```python
from build123d import *

# Parameters (mm, degrees)
SKETCH1_W           = 10
SKETCH1_H           = 10
BOSS_EXTRUDE1_DEPTH = 2
SKETCH2_R           = 1.55
SKETCH2_R_2         = 1.6
SKETCH2_R_3         = 0.5
SKETCH2_W           = 1.85
SKETCH2_H           = 1.85
SKETCH2_W_2         = 1.95
SKETCH2_H_2         = 1.95
SKETCH2_W_3         = 1.9
SKETCH2_H_3         = 1.9
CUT_EXTRUDE1_DEPTH  = 10
FILLET1_R           = 2


with BuildPart() as part:
    # Sketch1 → Boss-Extrude1 (new body)
    with BuildSketch(Plane(origin=(0, 0, 0), x_dir=(1, 0, 0), z_dir=(0, 1, 0))):
        with Locations((-46.016664058, -38.292528072)):
            Rectangle(SKETCH1_W, SKETCH1_H)
    extrude(amount=BOSS_EXTRUDE1_DEPTH)

    # Sketch2 → Cut-Extrude1 (cut)
    with BuildSketch(Plane(origin=(0, 2, 0), x_dir=(1, 0, 0), z_dir=(0, 1, 0))):
        with Locations(Location((-48.08551258, -40.164750495, 0), (0, 0, 270))):
            Circle(SKETCH2_R)
        with Locations(Location((-43.742640476, -40.164750495, 0), (0, 0, 270))):
            Circle(SKETCH2_R_2)
        with Locations(Location((-49.709815138, -37.736845618, 0), (0, 0, 270))):
            Circle(SKETCH2_R_3)
        with Locations((-48.955794355, -35.478207728)):
            Rectangle(SKETCH2_W, SKETCH2_H)
        with Locations((-43.041207223, -35.394011884)):
            Rectangle(SKETCH2_W_2, SKETCH2_H_2)
        with Locations((-46.016664058, -35.479919958)):
            Rectangle(SKETCH2_W_3, SKETCH2_H_3)
    extrude(amount=-CUT_EXTRUDE1_DEPTH, mode=Mode.SUBTRACT)

    # Fillet1
    fillet1_edges = [part.edges().sort_by_distance(p)[0] for p in [
        (-51.016664058, 1, 33.292528072),
        (-41.016664058, 1, 33.292528072),
        (-41.016664058, 1, 43.292528072),
        (-51.016664058, 1, 43.292528072),
    ]]
    fillet(fillet1_edges, radius=FILLET1_R)


solid = part.part
```
Geometry: final body of the model. Coordinates: model frame, mm. A direction names the side the tool comes from. Round coordinates to 2 decimals unless told otherwise and drop trailing zeros. Order: outer loops, then holes, each group sorted by start corner. A loop starts at its lowest first (then second) coordinate and runs counter-clockwise, first axis right, second up. Notation, with made-up numbers: (66.25, -39.75) - (118.25, -39.75) arc R32 ccw to (118.25, -0.75) - close; hole circle Ø10 at (86.5, 88). An arc over 180 degrees is marked (long way). Use CSV: the item, a comma, the result in double quotes. Start each with the question number.
Q1. Material intervals for line 1 along X through (y, z) = (1.55, 36); line 2 along Z through (x, y) = (-46.75, 0.7); line 3 along Z through (x, y) = (-43.5, 0.5), sorted ascending. Write a range as from..to.
Q2. Section query C-C (z = 37.5). Return loops of the section in (x, y), and give its area (3 significant figures).
Q3. Section query D-D (y = 0.6). Return loops of the section in (x, z), and give its area (3 significant figures).
Q4. Access query for faces 4 (the face through (-49, 1, 36.403)), 5 (the face through (-46, 0, 38)). Directions: +Z, -Z, +X, -X, +Y, -Y. A direction counts if a zero-diameter tool reaches every point of the face in a straight line with its end or side. Return the directions, or none.
Q5. Section query B-B (x = -50). Return loops of the section in (y, z).
Q6. Mould query, pull axis X, two halves, no side actions, for faces 1 (the face through (-41.618, 1.014, 42.722)), 2 (the face through (-43, 1, 36.369)), 3 (the face through (-46, 1, 43.293)). Classes: +X half, -X half, draft (parallel to the pull), parting line (faces both ways), or undercut.
Q7. Section query A-A (z = 35.5). Return loops of the section in (x, y), and give its area (3 significant figures).
Result set:
1,line 1,"x = -51.02..-49.88, -48.03..-46.97, -45.07..-44.02, -42.07..-41.02"
1,line 2,"z = 33.29..34.53, 36.43..39.38, 40.95..43.29"
1,line 3,"z = 33.29..34.42, 36.37..38.58, 41.75..43.29"
2,outline,"(-51.02, 0) - (-50.15, 0) - (-50.15, 2) - (-51.02, 2) - close; (-49.27, 0) - (-41.02, 0) - (-41.02, 2) - (-49.27, 2) - close"
2,area,"18.2 mm2"
3,outline,"(-51.02, 35.29) arc R2 ccw to (-49.02, 33.29) - (-43.02, 33.29) arc R2 ccw to (-41.02, 35.29) - (-41.02, 41.29) arc R2 ccw to (-43.02, 43.29) - (-49.02, 43.29) arc R2 ccw to (-51.02, 41.29) - close; hole circle Ø1 at (-49.71, 37.74); hole (-49.88, 34.55) - (-48.03, 34.55) - (-48.03, 36.4) - (-49.88, 36.4) - close; hole circle Ø3.1 at (-48.09, 40.16); hole (-46.97, 34.53) - (-45.07, 34.53) - (-45.07, 36.43) - (-46.97, 36.43) - close; hole circle Ø3.2 at (-43.74, 40.16); hole (-44.02, 34.42) - (-42.07, 34.42) - (-42.07, 36.37) - (-44.02, 36.37) - close"
3,area,"69.4 mm2"
4,face 4,"+Y, -Y"
4,face 5,"+Z, -Z, +X, -X, -Y"
5,outline,"(0, 33.55) - (2, 33.55) - (2, 37.33) - (0, 37.33) - close; (0, 38.14) - (2, 38.14) - (2, 43.03) - (0, 43.03) - close"
6,face 1,"+X half"
6,face 2,"undercut"
6,face 3,"draft"
7,outline,"(-51.02, 0) - (-49.88, 0) - (-49.88, 2) - (-51.02, 2) - close; (-48.03, 0) - (-46.97, 0) - (-46.97, 2) - (-48.03, 2) - close; (-45.07, 0) - (-44.02, 0) - (-44.02, 2) - (-45.07, 2) - close; (-42.07, 0) - (-41.02, 0) - (-41.02, 2) - (-42.07, 2) - close"
7,area,"8.60 mm2"
